Source: CAD feature listing. Evaluate the final solid. Frame: model axes, mm. Face numbers are marked on the shaded views. A direction names the side the tool comes from. Coordinates: 2 decimals unless noted, no trailing zeros. Order: outer loops, then holes, each group sorted by start corner. A loop starts at its lowest first (then second) coordinate and runs counter-clockwise, first axis right, second up. Notation, with made-up numbers: (75, 70) -> (82, 70) arc R9 cw to (82, 82) -> close; hole circle Ø11 at (54.25, 84.5). An arc over 180 degrees is marked (long way). Put each result on its own line as item: value.
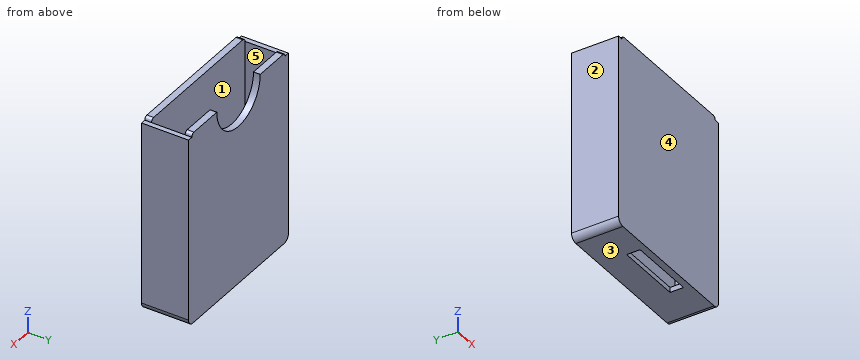
from build123d import *

# Parameters (mm, degrees)
BOSS_EXTRUDE23_DEPTH = 1
BOSS_EXTRUDE27_DEPTH = 6
BOSS_EXTRUDE28_START = 6
BOSS_EXTRUDE28_DEPTH = 1
CUT_EXTRUDE9_DEPTH   = 1
SKETCH15_W           = 10
SKETCH15_H           = 2
CUT_EXTRUDE11_DEPTH  = 10


with BuildPart() as part:
    # Sketch10 → Boss-Extrude23 (new body)
    with BuildSketch(Plane(origin=(0, 0, 0), x_dir=(1, 0, 0), z_dir=(0, 1, 0))):
        with BuildLine():
            Line((-11.5, -13.5), (-10.75, -13.5))
            ThreePointArc((-10.75, -13.5), (-10.603553391, -13.853553391), (-10.25, -14))
            Line((-10.25, -14), (10.25, -14))
            ThreePointArc((10.25, -14), (10.603553391, -13.853553391), (10.75, -13.5))
            Line((10.75, -13.5), (11.5, -13.5))
            Line((11.5, -13.5), (11.5, 13.75))
            ThreePointArc((11.5, 13.75), (11.207106781, 14.457106781), (10.5, 14.75))
            Line((10.5, 14.75), (-10.5, 14.75))
            ThreePointArc((-10.5, 14.75), (-11.207106781, 14.457106781), (-11.5, 13.75))
            Line((-11.5, 13.75), (-11.5, -13.5))
        make_face()
    extrude(amount=BOSS_EXTRUDE23_DEPTH)

    # Sketch10_6 → Boss-Extrude27 (add)
    with BuildSketch(Plane(origin=(0, 0, 0), x_dir=(1, 0, 0), z_dir=(0, 1, 0))):
        with BuildLine():
            Line((-11.5, -13.5), (-10.75, -13.5))
            Line((-10.75, -13.5), (-10.75, 13.5))
            ThreePointArc((-10.75, 13.5), (-10.603553391, 13.853553391), (-10.25, 14))
            Line((-10.25, 14), (10.25, 14))
            ThreePointArc((10.25, 14), (10.603553391, 13.853553391), (10.75, 13.5))
            Line((10.75, 13.5), (10.75, -13.5))
            Line((10.75, -13.5), (11.5, -13.5))
            Line((11.5, -13.5), (11.5, 13.75))
            ThreePointArc((11.5, 13.75), (11.207106781, 14.457106781), (10.5, 14.75))
            Line((10.5, 14.75), (4.75, 14.75))
            Line((4.75, 14.75), (-4.75, 14.75))
            Line((-4.75, 14.75), (-10.5, 14.75))
            ThreePointArc((-10.5, 14.75), (-11.207106781, 14.457106781), (-11.5, 13.75))
            Line((-11.5, 13.75), (-11.5, -13.5))
        make_face()
    extrude(amount=BOSS_EXTRUDE27_DEPTH)

    # Sketch10_7 → Boss-Extrude28 (add)
    with BuildSketch(Plane(origin=(0, 0, 0), x_dir=(1, 0, 0), z_dir=(0, 1, 0)).offset(BOSS_EXTRUDE28_START)):
        with BuildLine():
            Line((-11.5, -13.5), (-10.75, -13.5))
            Line((-10.75, -13.5), (-10.75, 13.5))
            ThreePointArc((-10.75, 13.5), (-10.603553391, 13.853553391), (-10.25, 14))
            Line((-10.25, 14), (10.25, 14))
            ThreePointArc((10.25, 14), (10.603553391, 13.853553391), (10.75, 13.5))
            Line((10.75, 13.5), (10.75, -13.5))
            Line((10.75, -13.5), (11.5, -13.5))
            Line((11.5, -13.5), (11.5, 13.75))
            ThreePointArc((11.5, 13.75), (11.207106781, 14.457106781), (10.5, 14.75))
            Line((10.5, 14.75), (4.75, 14.75))
            Line((4.75, 14.75), (-4.75, 14.75))
            Line((-4.75, 14.75), (-10.5, 14.75))
            ThreePointArc((-10.5, 14.75), (-11.207106781, 14.457106781), (-11.5, 13.75))
            Line((-11.5, 13.75), (-11.5, -13.5))
        make_face()
        with BuildLine():
            Line((10.75, 13.5), (10.75, -13.5))
            ThreePointArc((10.75, -13.5), (10.603553391, -13.853553391), (10.25, -14))
            Line((10.25, -14), (-10.25, -14))
            ThreePointArc((-10.25, -14), (-10.603553391, -13.853553391), (-10.75, -13.5))
            Line((-10.75, -13.5), (-10.75, 13.5))
            ThreePointArc((-10.75, 13.5), (-10.603553391, 13.853553391), (-10.25, 14))
            Line((-10.25, 14), (10.25, 14))
            ThreePointArc((10.25, 14), (10.603553391, 13.853553391), (10.75, 13.5))
        make_face()
    extrude(amount=BOSS_EXTRUDE28_DEPTH)

    # Sketch13 → Cut-Extrude9 (cut)
    with BuildSketch(Plane(origin=(0, 7, 0), x_dir=(1, 0, 0), z_dir=(0, 1, 0))):
        with BuildLine():
            Line((-5, -14), (5, -14))
            ThreePointArc((5, -14), (0, -9), (-5, -14))
        make_face()
    extrude(amount=-CUT_EXTRUDE9_DEPTH, mode=Mode.SUBTRACT)

    # Sketch15 → Cut-Extrude11 (cut)
    with BuildSketch(Plane(origin=(0, 0, -14.75), x_dir=(-1, 0, 0), z_dir=(0, 0, -1))):
        with Locations((0, 2)):
            Rectangle(SKETCH15_W, SKETCH15_H)
    extrude(amount=-CUT_EXTRUDE11_DEPTH, mode=Mode.SUBTRACT)


solid = part.part
1. Pull-direction query (X, two-part tool) for the marked faces 1, 2 and 3; classes: pulls with the +X half, pulls with the -X half, needs draft (parallel to the pull), parting line crosses it, or undercut.
Numbers:
face 1: undercut
face 2: pulls with the -X half
face 3: needs draft
2. Ray query, line 1 along X through (y, z) = (2.5, -6); line 2 along Y through (x, z) = (-3, 7); line 3 along Z through (x, y) = (7.5, 3.75). Return the intervals inside material, ascending.
Numbers:
line 1: x = -11.5 to -10.75, 10.75 to 11.5
line 2: y = 0 to 1, 6 to 7
line 3: z = -14.75 to -14
3. Cut plane A-A on x = 0. Output: boundary loops of the cut face in (y, z).
Numbers:
outline: (0, -14.75) -> (1, -14.75) -> (1, 14) -> (0, 14) -> close; (3, -14.75) -> (7, -14.75) -> (7, 9) -> (6, 9) -> (6, -14) -> (3, -14) -> close
4. First-contact query: pin 1 (0.8 mm diameter, centred on x = -11, y = 2.5, fed in from +Z); pin 2 (4 mm diameter, centred on x = 2.5, y = 4.5, fed in from +Z); pin 3 (4 mm diameter, centred on x = 1.5, y = 6, fed in from +Z). Flat tips, straight axial feed; report the tip coordinate or a pass-through.
Numbers:
pin 1: stops at z = 13.5
pin 2: stops at z = 10.78
pin 3: stops at z = 10.43
5. Cut plane C-C on z = -10. Output: boundary loops of the cut face in (x, y).
Numbers:
outline: (-11.5, 0) -> (11.5, 0) -> (11.5, 7) -> (-11.5, 7) -> close; hole (-10.75, 1) -> (10.75, 1) -> (10.75, 6) -> (-10.75, 6) -> close
6. Set-up query: the marked faces 4 and 5. Return all of +Z, -Z, +X, -X, +Y, -Y with unobstructed straight access to the full face (end or side cutting, diameter ignored); none if empty.
Numbers:
face 4: +Z, -Z, +X, -X, -Y
face 5: +Z
7. Cut plane D-D on y = 3.5. Output: boundary loops of the cut face in (x, z).
Numbers:
outline: (-11.5, -13.75) arc R1 ccw to (-10.5, -14.75) -> (10.5, -14.75) arc R1 ccw to (11.5, -13.75) -> (11.5, 13.5) -> (10.75, 13.5) -> (10.75, -13.5) arc R0.5 cw to (10.25, -14) -> (-10.25, -14) arc R0.5 cw to (-10.75, -13.5) -> (-10.75, 13.5) -> (-11.5, 13.5) -> close
8. Cut plane B-B on y = 1.5. Output: boundary loops of the cut face in (x, z).
Numbers:
outline: (-11.5, -13.75) arc R1 ccw to (-10.5, -14.75) -> (-5, -14.75) -> (-5, -14) -> (-10.25, -14) arc R0.5 cw to (-10.75, -13.5) -> (-10.75, 13.5) -> (-11.5, 13.5) -> close; (5, -14.75) -> (10.5, -14.75) arc R1 ccw to (11.5, -13.75) -> (11.5, 13.5) -> (10.75, 13.5) -> (10.75, -13.5) arc R0.5 cw to (10.25, -14) -> (5, -14) -> close
